Source: CAD feature listing. Evaluate the final solid. Frame: model axes, mm. A direction names the side the tool comes from. Round coordinates to 2 decimals unless told otherwise and drop trailing zeros. Loops run counter-clockwise (first coordinate to the right, second up) from the corner with the lowest first, then second, coordinate; pieces in that order, holes last.
(1) Material intervals for probe 1 along X at (y, z) = (11.05, 5.5); probe 2 along X at (y, z) = (10, -6.5); probe 3 along X at (y, z) = (-5.5, 4), sorted ascending.
(2) First-contact query: pin 1 Ø6.5 at (y, z) = (15.5, -3) entering from -X; pin 2 Ø0.6 at (y, z) = (19, 6.5) entering from +X; pin 3 Ø0.6 at (x, y) = (6, 18) entering from +Z (3 decimals); pin 4 Ø3 at (x, z) = (-24.2, 5.5) entering from +Y. Flat tips, straight axial feed; report the tip coordinate or a pass-through.
(3) Section A-A, the plane x = -24.2. Return the cut outline in (y, z).
(4) Mould query, pull axis Y, two halves, no side actions, for faces 1 (the flat face through (5, 18, 8.375)), 2 (the flat face through (-0.285, -16.402, 9.384)), 3 (the flat face through (-18, 17.5, 8)). Classes: pulls with the +Y half, pulls with the -Y half, needs draft (parallel to the pull), parting line crosses it, or undercut.
(5) Set-up query: faces 4 (the flat face through (-20.35, -3, 0)), 5 (the flat face through (5, 18, -8.375)), 6 (the flat face through (20.35, -3, 0)), 7 (the flat face through (24, 11.5, 0)), 8 (the cylindrical face through (-20.345, 18.437, -0.301)). Return all of +Z, -Z, +X, -X, +Y, -Y with unobstructed straight access to the full face (end or side cutting, diameter ignored); none if empty.
(6) Section C-C, the plane x = 11. Return the cut outline in (y, z) (3 decimals), plus the area to 3 significant figures.
(7) Section B-B, the plane z = -5.5. Count the separate pieces of the cut face and the enclosed holes in it, plus the area to 3 significant figures.
```python
from build123d import *

# Parameters (mm, degrees)
ESQUISSE1_W                = 40.7
ESQUISSE1_H                = 35
EXTRUSION1_DEPTH           = 10
ESQUISSE2_W                = 20
ESQUISSE2_H                = 2.4
EXTRUSION2_DEPTH           = 6.7
CHANFREIN1_SIZE            = 1.25
CHANFREIN1_SIZE2           = 2.165063509
EXTRUSION3_DEPTH           = 1.9
ESQUISSE4_R                = 6.425
EXTRUSION4_DEPTH           = 1.5
ESQUISSE5_R                = 2
EXTRUSION5_DEPTH           = 10
R_P_TITION_LIN_AIRE1_COUNT = 2
R_P_TITION_LIN_AIRE1_PITCH = 48.4
SYM_TRIE2_COPY_1_SKETCH_R  = 2
SYM_TRIE2_COPY_1_DEPTH     = 10
ESQUISSE6_R                = 2.9
EXTRUSION6_DEPTH           = 3.7


with BuildPart() as part:
    # Esquisse1 → Extrusion1 (new, symmetric)
    with BuildSketch(Plane.XY):
        Rectangle(ESQUISSE1_W, ESQUISSE1_H)
    extrude(amount=EXTRUSION1_DEPTH, both=True)

    # Esquisse2 → Extrusion2 (add)
    with BuildSketch(Plane.ZY.offset(20.35)):
        with Locations((0, 10.3)):
            Rectangle(ESQUISSE2_W, ESQUISSE2_H)
    extrusion2 = extrude(amount=EXTRUSION2_DEPTH)

    # Symétrie1: Extrusion2 across plane
    add(extrusion2.mirror(Plane(origin=(0, 0, 0), x_dir=(0, 0, 1), z_dir=(1, 0, 0))))

    # Chanfrein1
    chanfrein1_edges = [part.edges().sort_by_distance(p)[0] for p in [
        (-20.35, -17.5, 0),
        (0, -17.5, -10),
        (20.35, -17.5, 0),
        (0, -17.5, 10),
    ]]
    chanfrein1_side = [part.faces().sort_by_distance(p)[0] for p in [
        (0, -17.5, 0),
    ]]
    chamfer(chanfrein1_edges, length=CHANFREIN1_SIZE, length2=CHANFREIN1_SIZE2, reference=chanfrein1_side[0])

    # Esquisse3 → Extrusion3 (add)
    with BuildSketch(Plane(origin=(0, 17.5, 0), x_dir=(1, 0, 0), z_dir=(0, 1, 0))):
        with BuildLine():
            Line((-4.885626751, -8.375), (14.25, -8.375))
            Line((14.25, -8.375), (14.25, -3.464101615))
            ThreePointArc((14.25, -3.464101615), (16.25, 0), (14.25, 3.464101615))
            Line((14.25, 3.464101615), (14.25, 8.375))
            Line((14.25, 8.375), (-4.885626751, 8.375))
            ThreePointArc((-4.885626751, 8.375), (-20.35, 0), (-4.885626751, -8.375))
        make_face()
    extrude(amount=EXTRUSION3_DEPTH)

    # Esquisse4 → Extrusion4 (add)
    with BuildSketch(Plane(origin=(0, 19.4, 0), x_dir=(1, 0, 0), z_dir=(0, 1, 0))):
        with Locations(Location((-10.35, 0, 0), (0, 0, 270))):
            Circle(ESQUISSE4_R)
    extrude(amount=EXTRUSION4_DEPTH)

    # Esquisse5 → Extrusion5 (cut)
    with BuildSketch(Plane(origin=(0, 11.5, 0), x_dir=(1, 0, 0), z_dir=(0, 1, 0))):
        with Locations(Location((24.2, -5.5, 0), (0, 0, 270))):
            Circle(ESQUISSE5_R)
    extrusion5 = extrude(amount=-EXTRUSION5_DEPTH, mode=Mode.SUBTRACT)

    # Répétition linéaire1: Extrusion5 ×2
    with Locations(*[(-i * R_P_TITION_LIN_AIRE1_PITCH, 0, 0) for i in range(1, R_P_TITION_LIN_AIRE1_COUNT)]):
        add(extrusion5, mode=Mode.SUBTRACT)

    # Symétrie2: Extrusion5 across plane
    add(extrusion5.mirror(Plane.XY), mode=Mode.SUBTRACT)

    # Symétrie2 copy 1 sketch → Symétrie2 copy 1 (cut)
    with BuildSketch(Plane(origin=(-48.4, 11.5, 0), x_dir=(1, 0, 0), z_dir=(0, 1, 0))):
        with Locations((24.2, 5.5)):
            Circle(SYM_TRIE2_COPY_1_SKETCH_R)
    extrude(amount=-SYM_TRIE2_COPY_1_DEPTH, mode=Mode.SUBTRACT)

    # Esquisse6 → Extrusion6 (add)
    with BuildSketch(Plane(origin=(0, 20.9, 0), x_dir=(1, 0, 0), z_dir=(0, 1, 0))):
        with Locations(Location((-10.35, 0, 0), (0, 0, 270))):
            Circle(ESQUISSE6_R)
    extrude(amount=EXTRUSION6_DEPTH)


solid = part.part
```
Output values:
1. probe 1: x = -27.05 to -26.2, -22.2 to 22.2, 26.2 to 27.05
1. probe 2: x = -27.05 to -25.93, -22.47 to 22.47, 25.93 to 27.05
1. probe 3: x = -20.35 to 20.35
2. pin 1: stops at x = -20.35
2. pin 2: stops at x = 14.25
2. pin 3: stops at z = 8.375
2. pin 4: passes through
3. outline: (9.1, -10) - (11.5, -10) - (11.5, -7.5) - (9.1, -7.5) - close; (9.1, -3.5) - (11.5, -3.5) - (11.5, 3.5) - (9.1, 3.5) - close; (9.1, 7.5) - (11.5, 7.5) - (11.5, 10) - (9.1, 10) - close
4. face 1: needs draft
4. face 2: pulls with the -Y half
4. face 3: pulls with the +Y half
5. face 4: +Z, -Z, -X, -Y
5. face 5: -Z, +X, +Y
5. face 6: +Z, -Z, +X, -Y
5. face 7: +Z, -Z, +X, +Y
5. face 8: +Y
6. outline: (-17.5, -8.75) - (-15.335, -10) - (17.5, -10) - (17.5, -8.375) - (19.4, -8.375) - (19.4, 8.375) - (17.5, 8.375) - (17.5, 10) - (-15.335, 10) - (-17.5, 8.75) - close
6. area: 729 mm2
7. separate pieces: 3
7. enclosed holes: 0
7. area: 1,510 mm2
